```python
from build123d import *

# Parameters (mm, degrees)
SKETCH1_R           = 1.5
BOSS_EXTRUDE1_DEPTH = 3
CUT_EXTRUDE1_DEPTH  = 3
FILLET1_R           = 4


with BuildPart() as part:
    # Sketch1 → Boss-Extrude1 (new body)
    with BuildSketch(Plane(origin=(0, 0, 0), x_dir=(1, 0, 0), z_dir=(0, 1, 0))):
        with BuildLine():
            Line((0, 0), (-20, 0))
            ThreePointArc((-20, 0), (-22.828427125, 1.171572875), (-24, 4))
            Line((-24, 4), (-24, 7.0341572))
            ThreePointArc((-24, 7.0341572), (-23.888256641, 7.97301837), (-23.559269851, 8.85942379))
            Line((-23.559269851, 8.85942379), (-5.115247902, 44.82526659))
            ThreePointArc((-5.115247902, 44.82526659), (-3.641515588, 46.413287738), (-1.555978051, 47))
            Line((-1.555978051, 47), (1.555978051, 47))
            ThreePointArc((1.555978051, 47), (3.641515588, 46.413287738), (5.115247902, 44.82526659))
            Line((5.115247902, 44.82526659), (23.559269851, 8.85942379))
            ThreePointArc((23.559269851, 8.85942379), (23.888256641, 7.97301837), (24, 7.0341572))
            Line((24, 7.0341572), (24, 4))
            ThreePointArc((24, 4), (22.828427125, 1.171572875), (20, 0))
            Line((20, 0), (0, 0))
        make_face()
        with Locations((-16, 7)):
            Circle(SKETCH1_R, mode=Mode.SUBTRACT)
        with Locations((0, 41)):
            Circle(SKETCH1_R, mode=Mode.SUBTRACT)
        with Locations((16, 7)):
            Circle(SKETCH1_R, mode=Mode.SUBTRACT)
    extrude(amount=BOSS_EXTRUDE1_DEPTH)

    # Sketch2 → Cut-Extrude1 (cut)
    with BuildSketch(Plane(origin=(0, 3, 0), x_dir=(1, 0, 0), z_dir=(0, 1, 0))):
        with BuildLine():
            ThreePointArc((-12.990381057, 10.690853285), (0, 7.210091171), (12.990381057, 10.690853285))
            ThreePointArc((12.990381057, 10.690853285), (9.509618943, 23.681234342), (0, 33.190853285))
            ThreePointArc((0, 33.190853285), (-9.509618943, 23.681234342), (-12.990381057, 10.690853285))
        make_face()
    extrude(amount=-CUT_EXTRUDE1_DEPTH, mode=Mode.SUBTRACT)

    # Fillet1
    fillet1_edges = [part.edges().sort_by_distance(p)[0] for p in [
        (-12.990381057, 1.5, -10.690853285),
        (0, 1.5, -33.190853285),
        (12.990381057, 1.5, -10.690853285),
    ]]
    fillet(fillet1_edges, radius=FILLET1_R)


solid = part.part
```
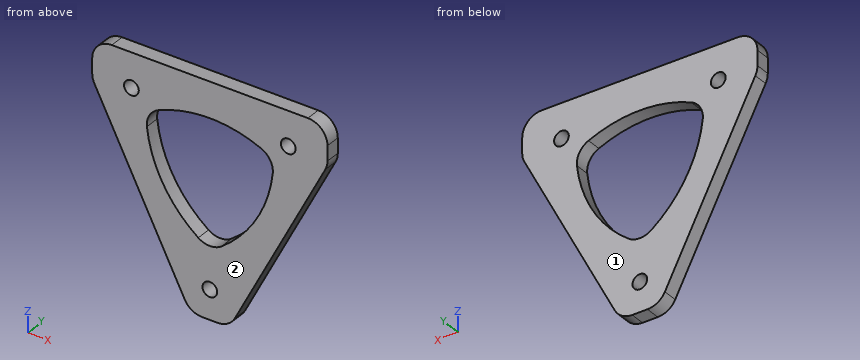
Check sheet for the modelled part. Datum: model origin and axes. Units: mm. Face numbers are marked on the shaded views. Coordinates: 2 decimals unless noted, no trailing zeros. Loops run counter-clockwise (first coordinate to the right, second up) from the corner with the lowest first, then second, coordinate; pieces in that order, holes last.
1) Sectioned sample at B-B (z = -21.5). Record the boundary of the cut face in (x, y).
2) Sectioned sample at A-A (x = 16). Record the boundary of the cut face in (y, z).
3) Material ranges on probe 1 along Z at (x, y) = (0, 1); probe 2 along X at (y, z) = (0.75, -7); probe 3 along X at (y, z) = (2.55, -6), recorded low to high.
4) Sectioned sample at C-C (y = 1). Count the separate pieces of the cut face and the enclosed holes in it, and give its area (3 significant figures).
5) Gauge pin test, flat end, axial feed: pin 1 (2.5 mm diameter, centred on x = 16, z = -7, fed in from -Y). Record the tip position at first contact, or that the pin passes through.
6) Release check for a two-part mould opening along Y. For the marked faces 1 and 2 record: released by +Y, released by -Y, zero draft, split by the parting line, or undercut.
Check sheet entries:
1. outline: (-17.08, 0) - (-10.64, 0) - (-10.64, 3) - (-17.08, 3) - close; (10.64, 0) - (17.08, 0) - (17.08, 3) - (10.64, 3) - close
2. outline: (0, -23.6) - (3, -23.6) - (3, -8.5) - (0, -8.5) - close; (0, -5.5) - (3, -5.5) - (3, 0) - (0, 0) - close
3. probe 1: z = -47 to -42.5, -39.5 to -32.42, -7.21 to 0
3. probe 2: x = -24 to -17.5, -14.5 to 14.5, 17.5 to 24
3. probe 3: x = -24 to -17.12, -14.88 to 14.88, 17.12 to 24
4. separate pieces: 1
4. enclosed holes: 4
4. area: 974 mm2
5. pin 1: passes through
6. face 1: released by +Y
6. face 2: released by -Y
